Input: part model. Units: mm. Frame: model coordinates. Face numbers are marked on the shaded views. Coordinates: 2 decimals unless noted, no trailing zeros. Write each loop counter-clockwise with the first axis right and the second up, starting at its lowest first coordinate (ties: lowest second). Pieces come first, ordered by that corner, then holes. Notation, with made-up numbers: (-10, 52) - (-5, 52) arc R21 cw to (-5, 89) - close; hole circle Ø3 at (12, 40.25). An arc over 180 degrees is marked (long way). Use CSV: the item, a comma, the result in double quotes.
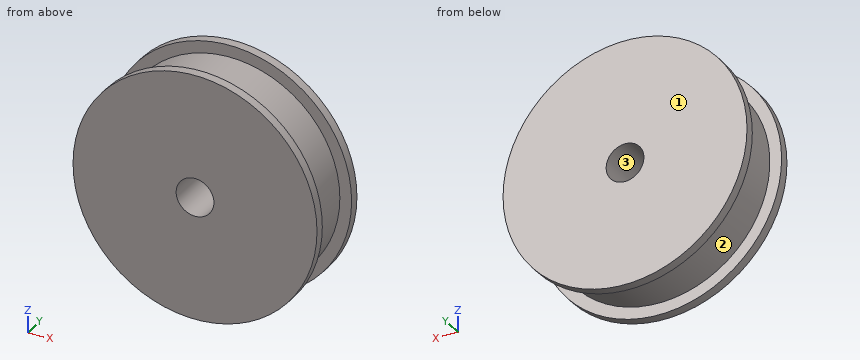
```python
from build123d import *

# Parameters (mm, degrees)
SKETCH_1_R          = 26
EXTRUDE_1_DEPTH     = 2
SKETCH_2_R          = 23.495
EXTRUDE_2_DEPTH     = 11
SKETCH_3_R          = 26
EXTRUDE_3_DEPTH     = 2
SKETCH_4_R          = 4.025
CUT_EXTRUDE_1_DEPTH = 16


with BuildPart() as part:
    # 草图1 → 凸台-拉伸1 (new body)
    with BuildSketch(Plane(origin=(0, 0, 0), x_dir=(1, 0, 0), z_dir=(0, 1, 0))):
        Circle(SKETCH_1_R)
    extrude(amount=EXTRUDE_1_DEPTH)

    # 草图2 → 凸台-拉伸2 (add)
    with BuildSketch(Plane(origin=(0, 2, 0), x_dir=(1, 0, 0), z_dir=(0, 1, 0))):
        Circle(SKETCH_2_R)
    extrude(amount=EXTRUDE_2_DEPTH)

    # 草图3 → 凸台-拉伸3 (add)
    with BuildSketch(Plane(origin=(0, 13, 0), x_dir=(1, 0, 0), z_dir=(0, 1, 0))):
        Circle(SKETCH_3_R)
    extrude(amount=EXTRUDE_3_DEPTH)

    # 草图4 → 切除-拉伸1 (cut, through all)
    with BuildSketch(Plane(origin=(0, 15, 0), x_dir=(1, 0, 0), z_dir=(0, 1, 0))):
        Circle(SKETCH_4_R)
    extrude(amount=-CUT_EXTRUDE_1_DEPTH, mode=Mode.SUBTRACT)


solid = part.part
```
(1) Draft query along Z for the marked faces 1, 2 and 3. Return one class per face: pulls with the +Z half, pulls with the -Z half, needs draft (parallel to the pull), parting line crosses it, or undercut.
Check values:
face 1,"needs draft"
face 2,"parting line crosses it"
face 3,"undercut"
(2) Cut plane C-C on y = 13.75. Return loops of the section in (x, z) (3 decimals).
Check values:
outline,"circle Ø52 at (0, 0); hole circle Ø8.05 at (0, 0)"
(3) Cut plane A-A on z = 0. Return loops of the section in (x, y) (3 decimals), and give its area (3 significant figures).
Check values:
outline,"(-26, 0) - (-4.025, 0) - (-4.025, 15) - (-26, 15) - (-26, 13) - (-23.495, 13) - (-23.495, 2) - (-26, 2) - close; (4.025, 0) - (26, 0) - (26, 2) - (23.495, 2) - (23.495, 13) - (26, 13) - (26, 15) - (4.025, 15) - close"
area,"604 mm^2"
(4) Cut plane D-D on x = 13.5. Return loops of the section in (y, z).
Check values:
outline,"(0, -22.22) - (2, -22.22) - (2, -19.23) - (13, -19.23) - (13, -22.22) - (15, -22.22) - (15, 22.22) - (13, 22.22) - (13, 19.23) - (2, 19.23) - (2, 22.22) - (0, 22.22) - close"
(5) Ray query, probe 1 along X at (y, z) = (5.75, 0) (3 decimals); probe 2 along Y at (x, z) = (-22.5, -7). Return the intervals inside material, ascending. Write a range as from..to.
Check values:
probe 1,"-23.495..-4.025, 4.025..23.495"
probe 2,"0..2, 13..15"
(6) Pin query (flat end, axial travel): pin 1 Ø2 at (x, y) = (-3.5, 6.5) entering from +Z; pin 2 Ø6 at (x, y) = (0.5, 6) entering from +Z (3 decimals); pin 3 Ø8 at (y, z) = (7, -12) entering from -X. Return the tip coordinate at first contact, or that it passes through.
Check values:
pin 1,"z = 23.36"
pin 2,"z = 23.495"
pin 3,"x = -22.09"
(7) Cut plane B-B on x = 0. Return loops of the section in (y, z) (3 decimals).
Check values:
outline,"(0, -26) - (2, -26) - (2, -23.495) - (13, -23.495) - (13, -26) - (15, -26) - (15, -4.025) - (0, -4.025) - close; (0, 4.025) - (15, 4.025) - (15, 26) - (13, 26) - (13, 23.495) - (2, 23.495) - (2, 26) - (0, 26) - close"
